Could you check a few things on this drawing? It's one solid part, dimensions in mm from its lowest x, y, z. A direction names the side the tool comes from. Coordinates: 2 decimals unless noted, no trailing zeros. Write each loop counter-clockwise with the first axis right and the second up, starting at its lowest first coordinate (ties: lowest second). Pieces come first, ordered by that corner, then holes. Notation, with made-up numbers: M -25.75,2.25 L -14.75,2.25 A17 cw -14.75,24.25 Z; hole C -39.5,-39 d6. An arc over 180 degrees is marked long. Use a Markdown table: item, result.
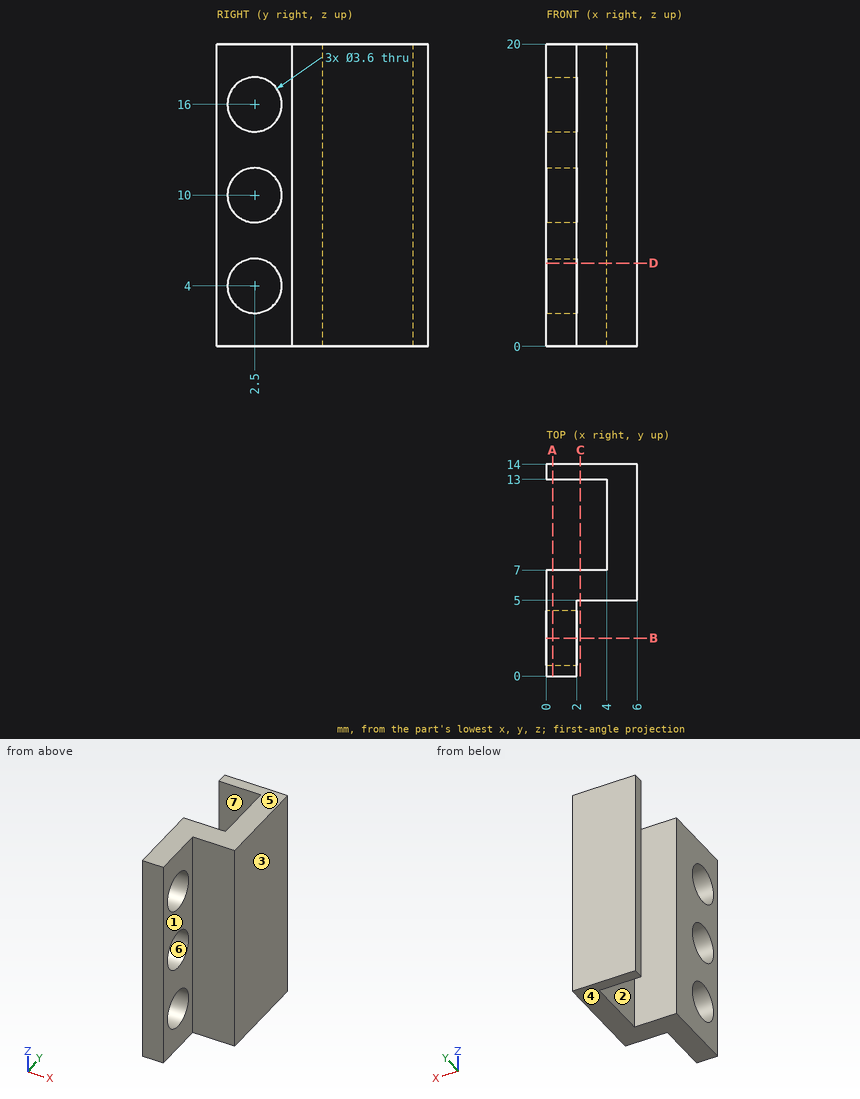
1. Suppose I cut it at B-B on y = 2.5. Write out the boundary of the cut face in (x, z), and give its area (3 significant figures).
Answers follow:
| item | result |
|---|---|
| outline | M 0,0 L 2,0 L 2,2.2 L 0,2.2 Z; M 0,5.8 L 2,5.8 L 2,8.2 L 0,8.2 Z; M 0,11.8 L 2,11.8 L 2,14.2 L 0,14.2 Z; M 0,17.8 L 2,17.8 L 2,20 L 0,20 Z |
| area | 18.4 mm2 |
2. Suppose I cut it at C-C on x = 2.25. Write out the boundary of the cut face in (y, z), and give its area (3 significant figures).
Answers follow:
| item | result |
|---|---|
| outline | M 5,0 L 7,0 L 7,20 L 5,20 Z; M 13,0 L 14,0 L 14,20 L 13,20 Z |
| area | 60.0 mm2 |
3. Will these pins go through, and if not, where does the flat tip stop? pin 1 Ø1.2 at (x, z) = (3, 5) entering from -Y; pin 2 Ø6 at (y, z) = (2.5, 16) entering from -X; pin 3 Ø1.5 at (y, z) = (3.5, 11.5) entering from +X; pin 4 Ø1.8 at (y, z) = (10.5, 6.5) entering from -X.
Answers follow:
| item | result |
|---|---|
| pin 1 | stops at y = 5 |
| pin 2 | stops at x = 0 |
| pin 3 | stops at x = 2 |
| pin 4 | stops at x = 4 |
4. Suppose I cut it at D-D on z = 5.5. Write out the boundary of the cut face in (x, y).
Answers follow:
| item | result |
|---|---|
| outline | M 0,0 L 2,0 L 2,1.51 L 0,1.51 Z; M 0,3.49 L 2,3.49 L 2,5 L 6,5 L 6,14 L 0,14 L 0,13 L 4,13 L 4,7 L 0,7 Z |
5. I need wall thicknesses on probe 1 along Z at (x, y) = (1.25, 2.5); probe 2 along Z at (x, y) = (1.9, 4); probe 3 along Y at (x, z) = (2.1, 1). Which ranges of each line are inside material? Lowest first, please.
Answers follow:
| item | result |
|---|---|
| probe 1 | z = 0 to 2.2, 5.8 to 8.2, 11.8 to 14.2, 17.8 to 20 |
| probe 2 | z = 0 to 3.01, 4.99 to 9.01, 10.99 to 15.01, 16.99 to 20 |
| probe 3 | y = 5 to 7, 13 to 14 |
6. Which directions (+Z, -Z, +X, -X, +Y, -Y) give clear straight access to the entire face, cutting with the end or side of a thin tool? Please do the marked faces 1, 2 and 3.
Answers follow:
| item | result |
|---|---|
| face 1 | +Z, -Z, +X, -Y |
| face 2 | +Z, -Z, -X |
| face 3 | +Z, -Z, +X, +Y, -Y |
7. Suppose I cut it at A-A on x = 0.4. Write out the boundary of the cut face in (y, z).
Answers follow:
| item | result |
|---|---|
| outline | M 0,0 L 7,0 L 7,20 L 0,20 Z; M 13,0 L 14,0 L 14,20 L 13,20 Z; hole C 2.5,4 d3.6; hole C 2.5,10 d3.6; hole C 2.5,16 d3.6 |
8. We'd pull the mould along Z, two halves only. Please class the marked faces 4, 5, 6 and 7: +Z half, -Z half, draft (parallel to the pull), parting line (faces both ways), or undercut.
Answers follow:
| item | result |
|---|---|
| face 4 | -Z half |
| face 5 | +Z half |
| face 6 | undercut |
| face 7 | draft |
